Study the drawing (mm; zero at the part's minimum x, y, z) and answer. A direction names the side the tool comes from. Coordinates: 2 decimals unless noted, no trailing zeros. Order: outer loops, then holes, each group sorted by start corner. A loop starts at its lowest first (then second) coordinate and runs counter-clockwise, first axis right, second up. Notation, with made-up numbers: M 88,0 L 132,0 A11 ccw 132,7 Z; hole C 7.25,-13 d2. An arc over 180 degrees is marked long. One line per item, written item: value. Start each with the question number.
Q1. For the marked faces 5, 6 and 7, determine the directions among +Z, -Z, +X, -X, +Y, -Y from which every point of the face is accessible in a straight line to the end or side of a thin tool.
Q2. Straight lines are drawn through the part: line 1 along X through (y, z) = (5.25, 1.2) (1 decimal); line 2 along X through (y, z) = (5, 0.4) (1 decimal); line 3 along Y through (x, z) = (5.5, 0.4) (1 decimal). For each, find the intervals that lie inside material, in ascending order. Write a range as [from, to].
Q3. Each of these flat-tipped pins is pushed along its axis until it touches: pin 1 Ø0.8 at (x, z) = (0.5, 1) entering from +Y; pin 2 Ø0.8 at (x, z) = (9, 1) entering from -Y (1 decimal). Where does it stop, or does it pass through?
Q4. Determine the mould class of the marked faces 1, 2, 3 and 4 for opening direction X: pulls with the +X half, pulls with the -X half, needs draft (parallel to the pull), parting line crosses it, or undercut.
Q5. The part is cut by section D-D on y = 2.25. Give the vertices of the cut face in (x, z).
Q6. The part is cut by section C-C on y = 3.75. Give the vertices of the cut face in (x, z), then the cut area to 3 significant figures.
Q7. The part is cut by section B-B on x = 8.25. Give the vertices of the cut face in (y, z).
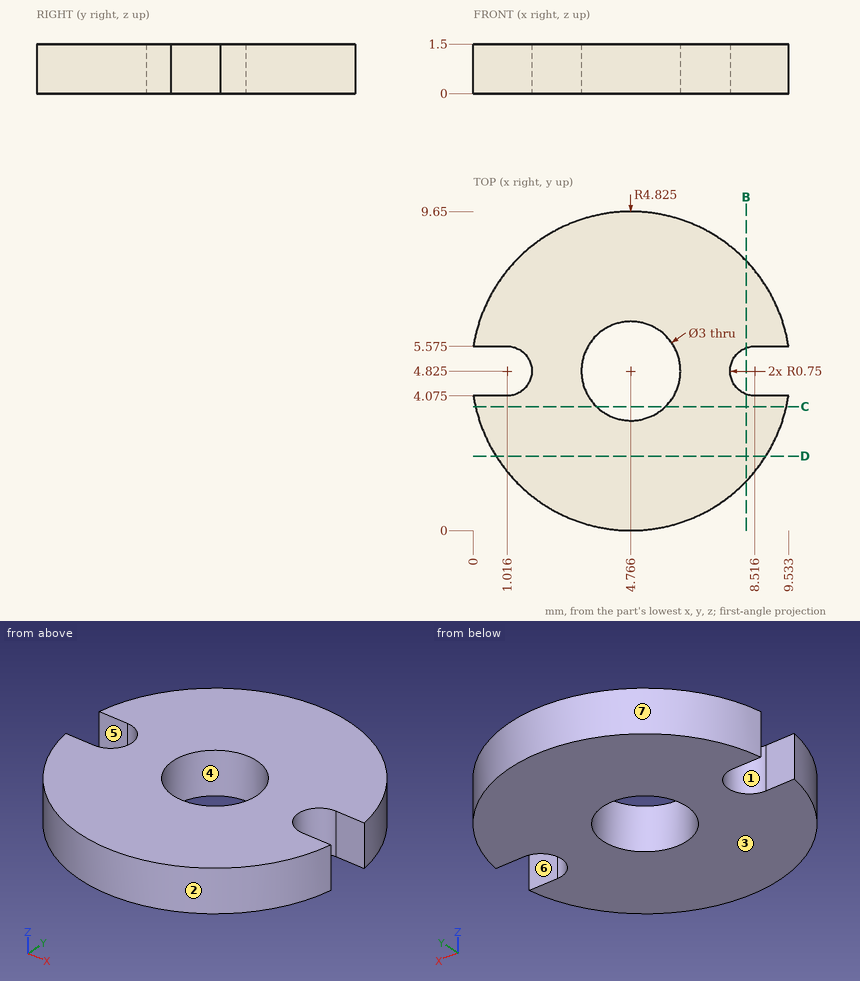
Output:
1. face 5: +Z, -Z, -X
1. face 6: +Z, -Z, +X
1. face 7: +Z, -Z, +Y
2. line 1: x = [1.6, 3.3], [6.2, 7.9]
2. line 2: x = [1.7, 3.3], [6.3, 7.8]
2. line 3: y = [0.1, 3.5], [6.1, 9.6]
3. pin 1: stops at y = 7.71
3. pin 2: stops at y = 1.9
4. face 1: pulls with the -X half
4. face 2: parting line crosses it
4. face 3: needs draft
4. face 4: undercut
5. outline: M 0.69,0 L 8.85,0 L 8.85,1.5 L 0.69,1.5 Z
6. outline: M 0.06,0 L 3.72,0 L 3.72,1.5 L 0.06,1.5 Z; M 5.81,0 L 9.47,0 L 9.47,1.5 L 5.81,1.5 Z
6. area: 11.0 mm^2
7. outline: M 1.49,0 L 4.12,0 L 4.12,1.5 L 1.49,1.5 Z; M 5.53,0 L 8.16,0 L 8.16,1.5 L 5.53,1.5 Z
